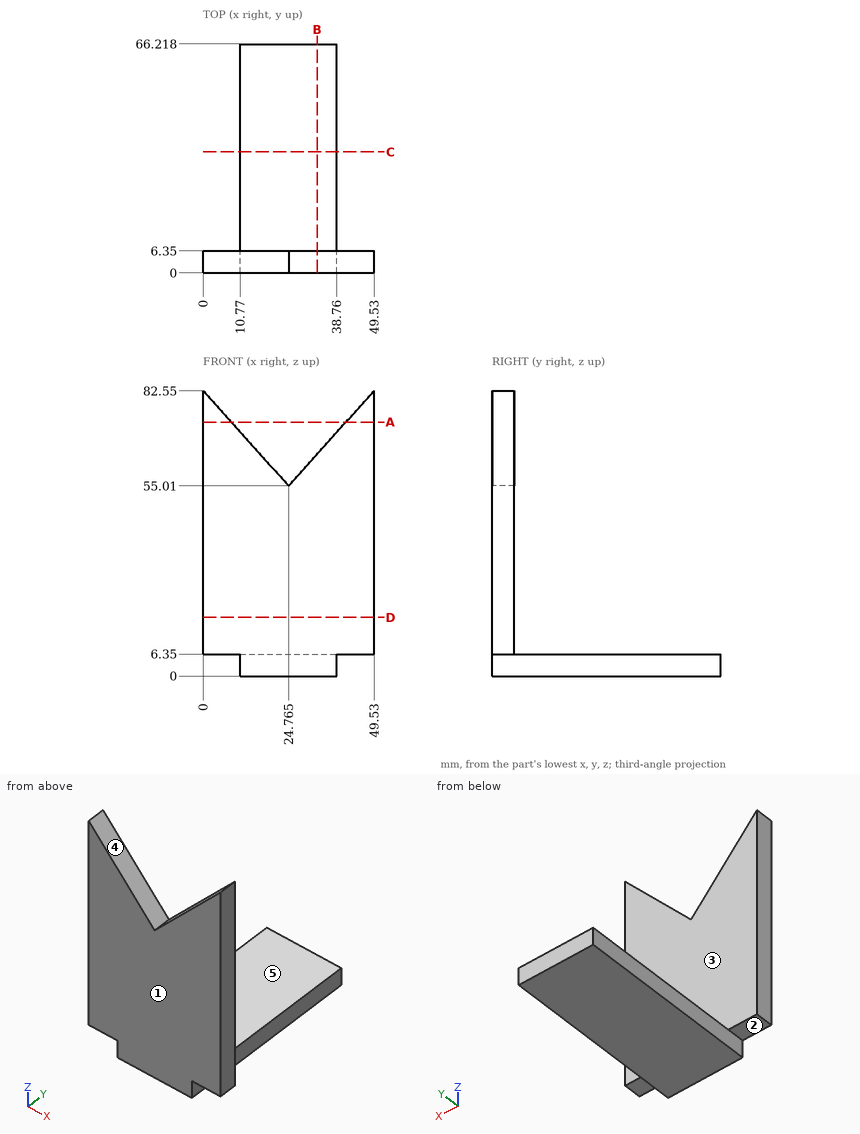
Could you check a few things on this drawing? It's one solid part, dimensions in mm from its lowest x, y, z. A direction names the side the tool comes from. Coordinates: 2 decimals unless noted, no trailing zeros. Loops run counter-clockwise (first coordinate to the right, second up) from the corner with the lowest first, then second, coordinate; pieces in that order, holes last. Notation, with made-up numbers: (-33.5, 52.25) - (-20.5, 52.25) arc R18 ccw to (-20.5, 67.25) - close; hole circle Ø9 at (-34.5, -27). An arc over 180 degrees is marked (long way). Answer as a JSON object with one key per item and string values. Group by question number.
Item 1: If we section it at C-C (y = 35): List the corners of the cut face in (x, z) for me, plus the area to 3 significant figures.
Item 2: If we mould it in two halves opening along X, with no side actions, what happens to the marked faces 4 and 5? For each: released by +X, released by -X, zero draft, split by the parting line, or undercut.
Item 3: If I drill on L1, parallel to Y at x = 30, z = 40, over which ranges is the centre line in solid material (lowest first)? Write a range as from..to.
Item 4: For pin 1 (10 mm diameter, centred on x = 36, z = 68, fed in from +Y); pin 2 (3 mm diameter, centred on y = 46.5, z = 2, fed in from +X); pin 3 (3 mm diameter, centred on x = 3.5, y = 4, fed in from -Z), each with a flat end and sliding along its axis, tell me the tip position at first contact or that it passes through.
Item 5: If we section it at A-A (z = 73.5): List the corners of the cut face in (x, y) for me, plus the area to 3 significant figures.
Item 6: If we section it at B-B (x = 33): List the corners of the cut face in (y, z) for me.
Item 7: On a 3-axis mill with a long thin cutter (end or side, diameter ignored), from which of +Z, -Z, +X, -X, +Y, -Y can I reach the whole of each face in a straight line? I mean the marked faces 1, 2 and 3. Say none if no direction works.
Item 8: If we section it at D-D (z = 17): List the corners of the cut face in (x, y) for me.
Returned:
{
 "1": {"outline": "(10.77, 0) - (38.76, 0) - (38.76, 6.35) - (10.77, 6.35) - close", "area": "178 mm²"},
 "2": {"face 4": "undercut", "face 5": "zero draft"},
 "3": {"L1": "y = 0..6.35"},
 "4": {"pin 1": "stops at y = 6.35", "pin 2": "stops at x = 38.76", "pin 3": "stops at z = 6.35"},
 "5": {"outline": "(0, 0) - (8.14, 0) - (8.14, 6.35) - (0, 6.35) - close; (41.39, 0) - (49.53, 0) - (49.53, 6.35) - (41.39, 6.35) - close", "area": "103 mm²"},
 "6": {"outline": "(0, 0) - (66.22, 0) - (66.22, 6.35) - (6.35, 6.35) - (6.35, 64.17) - (0, 64.17) - close"},
 "7": {"face 1": "+Z, -Z, +X, -X, -Y", "face 2": "-Z, -X, +Y, -Y", "face 3": "+Z, +X, -X, +Y"},
 "8": {"outline": "(0, 0) - (49.53, 0) - (49.53, 6.35) - (0, 6.35) - close"}
}
